```python
from build123d import *

# Parameters (mm, degrees)
SKETCH1_W           = 0.2
SKETCH1_H           = 3
SKETCH1_W_2         = 82.6
SKETCH1_H_2         = 100
BOSS_EXTRUDE1_DEPTH = 2.23


with BuildPart() as part:
    # Sketch1 → Boss-Extrude1 (new body)
    with BuildSketch(Plane(origin=(0, 0, 0), x_dir=(1, 0, 0), z_dir=(0, 1, 0))):
        with BuildLine():
            Line((43.1, -37.85), (43.1, -38.5))
            ThreePointArc((43.1, -38.5), (44.922195524, -38.020142239), (46.5, -36.99))
            Line((46.5, -36.99), (46.5, -35.49))
            Line((46.5, -35.49), (43.1, -35.49))
            Line((43.1, -35.49), (43.1, -37.85))
        make_face()
        Polygon((41.5, -35.49), (41.3, -35.49), (41.3, -37.85), (43.1, -37.85), (43.1, -35.49), align=None)
        Polygon((45, -29.99), (41.3, -29.99), (41.3, -32.49), (41.5, -32.49), (46.5, -32.49), (46.5, -30.99), align=None)
        with Locations((41.4, -33.99)):
            Rectangle(SKETCH1_W, SKETCH1_H)
        Rectangle(SKETCH1_W_2, SKETCH1_H_2)
        Polygon((46.5, 42.51), (41.5, 42.51), (41.3, 42.51), (41.3, 40.01), (45, 40.01), (46.5, 41.01), align=None)
        with Locations((41.4, 44.01)):
            Rectangle(SKETCH1_W, SKETCH1_H)
        Polygon((41.5, 45.51), (43.1, 45.51), (43.1, 47.87), (41.3, 47.87), (41.3, 45.51), align=None)
        with BuildLine():
            ThreePointArc((43.1, 48.52), (44.922195524, 48.040142239), (46.5, 47.01))
            Line((46.5, 47.01), (46.5, 45.51))
            Line((46.5, 45.51), (43.1, 45.51))
            Line((43.1, 45.51), (43.1, 47.87))
            Line((43.1, 47.87), (43.1, 48.52))
        make_face()
        with BuildLine():
            Line((-43.1, -47.87), (-41.3, -47.87))
            Line((-41.3, -47.87), (-41.3, -45.51))
            Line((-41.3, -45.51), (-41.5, -45.51))
            Line((-41.5, -45.51), (-46.5, -45.51))
            Line((-46.5, -45.51), (-46.5, -47.01))
            ThreePointArc((-46.5, -47.01), (-44.922195524, -48.040142239), (-43.1, -48.52))
            Line((-43.1, -48.52), (-43.1, -47.87))
        make_face()
        Polygon((-41.3, -45.51), (-41.3, -40.01), (-45, -40.01), (-46.5, -41.01), (-46.5, -42.51), (-41.5, -42.51), (-41.5, -45.51), align=None)
        Polygon((-41.3, 29.99), (-41.3, 35.49), (-41.5, 35.49), (-41.5, 32.49), (-46.5, 32.49), (-46.5, 30.99), (-45, 29.99), align=None)
        with BuildLine():
            Line((-41.3, 35.49), (-41.3, 37.85))
            Line((-41.3, 37.85), (-43.1, 37.85))
            Line((-43.1, 37.85), (-43.1, 38.5))
            ThreePointArc((-43.1, 38.5), (-44.922195524, 38.020142239), (-46.5, 36.99))
            Line((-46.5, 36.99), (-46.5, 35.49))
            Line((-46.5, 35.49), (-41.5, 35.49))
            Line((-41.5, 35.49), (-41.3, 35.49))
        make_face()
    extrude(amount=BOSS_EXTRUDE1_DEPTH)


solid = part.part
```
Read the model definition and answer for the solid it produces. Units are mm, in the model's axes. A direction names the side the tool comes from. Give positions to 0.01 mm unless a question says otherwise; leave off trailing zeros. Write each loop counter-clockwise with the first axis right and the second up, starting at its lowest first coordinate (ties: lowest second). Pieces come first, ordered by that corner, then holes. Notation, with made-up numbers: M -31,45 L 19,45 A29 cw 19,84 Z; hole C -38,-24.5 d11. An arc over 180 degrees is marked long. Put each result on its own line as item: value. Start each with the question number.
1. Which of the six approach directions +Z, -Z, +X, -X, +Y, -Y give full straight-line access (tool end or side, diameter ignored) to faces 1 (the flat face through (-44, 1, -35.49)), 2 (the cylindrical face through (44.9, 1.1, 38.03)), 3 (the flat face through (44, 1, 32.49))?
2. Consider line 1 along X through (y, z) = (1.2, 14); line 2 along X through (y, z) = (1.7, -45). Determine where each line is inside the solid, lowest interval first.
3. Each of these flat-tipped pins is pushed along its axis until it touches: pin 1 Ø0.7 at (y, z) = (1, 1.5) entering from +X; pin 2 Ø0.7 at (x, y) = (-42, 1.5) entering from -Z; pin 3 Ø0.7 at (y, z) = (0.5, -46.5) entering from -X. Where does it stop, or does it pass through?
4. The part is cut by section A-A, the plane z = -6. Give the vertices of the cut face in (x, y).
5. For a pull along X with two mould halves and no side action, classify faces 4 (the flat face through (-41.3, 1, 49)), 5 (the flat face through (41.3, 1, -5)), 6 (the flat face through (-41.3, 1, 5)) as released by +X, released by -X, zero draft, split by the parting line, or undercut.
Final values:
1. face 1: -X, +Y, -Y
1. face 2: +Z, +X, +Y, -Y
1. face 3: +X, +Y, -Y
2. line 1: x = -41.3 to 41.3
2. line 2: x = -41.3 to 41.5
3. pin 1: stops at x = 41.3
3. pin 2: stops at z = -37.85
3. pin 3: stops at x = -41.3
4. outline: M -41.3,0 L 41.3,0 L 41.3,2.23 L -41.3,2.23 Z
5. face 4: undercut
5. face 5: released by +X
5. face 6: released by -X
